Geometry check sheet. Reference: the model listing, model coordinates, mm. A direction names the side the tool comes from. Round coordinates to 2 decimals unless told otherwise and drop trailing zeros. Write each loop counter-clockwise with the first axis right and the second up, starting at its lowest first coordinate (ties: lowest second). Pieces come first, ordered by that corner, then holes. Notation, with made-up numbers: (50.25, 55) -> (82.25, 55) arc R21 ccw to (82.25, 79) -> close; hole circle Ø1 at (87.5, -33). An arc over 180 degrees is marked (long way). Use a Markdown table: item, result.
```python
from build123d import *

# Parameters (mm, degrees)
CROQUIS1_W              = 36
CROQUIS1_H              = 36
SALIENTE_EXTRUIR1_DEPTH = 4
CROQUIS2_R              = 1.7
CORTAR_EXTRUIR1_DEPTH   = 6
CROQUIS3_R              = 3.1
CORTAR_EXTRUIR2_DEPTH   = 3.5
CROQUIS4_R              = 1.1
CORTAR_EXTRUIR3_DEPTH   = 6


with BuildPart() as part:
    # Croquis1 → Saliente-Extruir1 (new body)
    with BuildSketch(Plane(origin=(-12.9, 0, 0), x_dir=(0, 0, -1), z_dir=(1, 0, 0))):
        with Locations((-94.5, 0)):
            Rectangle(CROQUIS1_W, CROQUIS1_H)
    extrude(amount=SALIENTE_EXTRUIR1_DEPTH)

    # Croquis2 → Cortar-Extruir1 (cut)
    with BuildSketch(Plane(origin=(-13.9, 0, 0), x_dir=(0, 0, -1), z_dir=(1, 0, 0))):
        with Locations((-80.7, -13.85)):
            Circle(CROQUIS2_R)
        with Locations((-108.4, -13.85)):
            Circle(CROQUIS2_R)
        with Locations((-80.7, 13.85)):
            Circle(CROQUIS2_R)
        with Locations((-108.4, 13.85)):
            Circle(CROQUIS2_R)
    extrude(amount=CORTAR_EXTRUIR1_DEPTH, mode=Mode.SUBTRACT)

    # Croquis3 → Cortar-Extruir2 (cut)
    with BuildSketch(Plane(origin=(-13.9, 0, 0), x_dir=(0, 0, -1), z_dir=(1, 0, 0))):
        with Locations((-80.7, -13.85)):
            Circle(CROQUIS3_R)
        with Locations((-108.4, -13.85)):
            Circle(CROQUIS3_R)
        with Locations((-80.7, 13.85)):
            Circle(CROQUIS3_R)
        with Locations((-108.4, 13.85)):
            Circle(CROQUIS3_R)
    extrude(amount=CORTAR_EXTRUIR2_DEPTH, mode=Mode.SUBTRACT)

    # Croquis4 → Cortar-Extruir3 (cut)
    with BuildSketch(Plane(origin=(-13.9, 0, 0), x_dir=(0, 0, -1), z_dir=(1, 0, 0))):
        with Locations((-97, -10.5)):
            Circle(CROQUIS4_R)
        with Locations((-84.5, -10.5)):
            Circle(CROQUIS4_R)
        with Locations((-97, 10.5)):
            Circle(CROQUIS4_R)
        with Locations((-84.5, 10.5)):
            Circle(CROQUIS4_R)
    extrude(amount=CORTAR_EXTRUIR3_DEPTH, mode=Mode.SUBTRACT)


solid = part.part
```
(1) Section check A-A on z = 108.4. Record the cut outline in (x, y), plus the area to 3 significant figures.
A:
| item | result |
|---|---|
| outline | (-12.9, -18) -> (-8.9, -18) -> (-8.9, -15.55) -> (-10.4, -15.55) -> (-10.4, -16.95) -> (-12.9, -16.95) -> close; (-12.9, -10.75) -> (-10.4, -10.75) -> (-10.4, -12.15) -> (-8.9, -12.15) -> (-8.9, 12.15) -> (-10.4, 12.15) -> (-10.4, 10.75) -> (-12.9, 10.75) -> close; (-12.9, 16.95) -> (-10.4, 16.95) -> (-10.4, 15.55) -> (-8.9, 15.55) -> (-8.9, 18) -> (-12.9, 18) -> close |
| area | 103 mm2 |
(2) Access from +Z, -Z, +X, -X, +Y, -Y to the whole of each face (thin tool, end or side, straight path). Record for faces 1 (the face through (-11.67, -11.75, 82.98)), 2 (the face through (-10.9, 10.5, 85.6)).
A:
| item | result |
|---|---|
| face 1 | -X |
| face 2 | +X, -X |
(3) Section check D-D on z = 84.5. Record the cut outline in (x, y).
A:
| item | result |
|---|---|
| outline | (-12.9, -18) -> (-8.9, -18) -> (-8.9, -11.6) -> (-12.9, -11.6) -> close; (-12.9, -9.4) -> (-8.9, -9.4) -> (-8.9, 9.4) -> (-12.9, 9.4) -> close; (-12.9, 11.6) -> (-8.9, 11.6) -> (-8.9, 18) -> (-12.9, 18) -> close |
(4) Release check for a two-part mould opening along Y. For faces 3 (the face through (-11, -18, 95)), 4 (the face through (-11, 18, 95)), 5 (the face through (-11, 0, 112.5)), 6 (the face through (-9.66, 13.2, 106.83)) record: +Y half, -Y half, draft (parallel to the pull), parting line (faces both ways), or undercut.
A:
| item | result |
|---|---|
| face 3 | -Y half |
| face 4 | +Y half |
| face 5 | draft |
| face 6 | undercut |
(5) Thickness scan on line 1 (Y direction, x = -10.2, z = 84.5); line 2 (Y direction, x = -11.25, z = 108.4); line 3 (Z direction, x = -9.8, y = -13.85). Record the ranges inside material, lowest first.
A:
| item | result |
|---|---|
| line 1 | y = -18 to -11.6, -9.4 to 9.4, 11.6 to 18 |
| line 2 | y = -18 to -16.95, -10.75 to 10.75, 16.95 to 18 |
| line 3 | z = 76.5 to 79, 82.4 to 106.7, 110.1 to 112.5 |
(6) Section check B-B on y = 13.85. Record the cut outline in (x, z), plus the area to 3 significant figures.
A:
| item | result |
|---|---|
| outline | (-12.9, 76.5) -> (-8.9, 76.5) -> (-8.9, 79) -> (-10.4, 79) -> (-10.4, 77.6) -> (-12.9, 77.6) -> close; (-12.9, 83.8) -> (-10.4, 83.8) -> (-10.4, 82.4) -> (-8.9, 82.4) -> (-8.9, 106.7) -> (-10.4, 106.7) -> (-10.4, 105.3) -> (-12.9, 105.3) -> close; (-12.9, 111.5) -> (-10.4, 111.5) -> (-10.4, 110.1) -> (-8.9, 110.1) -> (-8.9, 112.5) -> (-12.9, 112.5) -> close |
| area | 103 mm2 |
(7) Section check C-C on x = -9.4. State how many separate pieces and enclosed holes the cut face has, plus the area to 3 significant figures.
A:
| item | result |
|---|---|
| separate pieces | 1 |
| enclosed holes | 8 |
| area | 1,240 mm2 |
(8) Gauge pin test, flat end, axial feed: pin 1 Ø1.9 at (y, z) = (13.5, 109.5) entering from -X. Record the tip position at first contact, or that the pin passes through.
A:
| item | result |
|---|---|
| pin 1 | stops at x = -10.4 |
